Read the model definition and answer for the solid it produces. Units are mm, in the model's axes. A direction names the side the tool comes from. Coordinates: 2 decimals unless noted, no trailing zeros. Order: outer loops, then holes, each group sorted by start corner. A loop starts at its lowest first (then second) coordinate and runs counter-clockwise, first axis right, second up. Notation, with made-up numbers: (3.5, 44.5) - (39.5, 44.5) arc R15 ccw to (39.5, 48.5) - close; hole circle Ø9 at (76.5, 46). An arc over 180 degrees is marked (long way). Use one line per item in the form item = value.
```python
from build123d import *

# Parameters (mm, degrees)
SKETCH1_W           = 25.4
SKETCH1_H           = 25.4
BOSS_EXTRUDE1_DEPTH = 114.3
SKETCH3_W           = 22.098
SKETCH3_H           = 22.098
CUT_EXTRUDE1_DEPTH  = 130.139939168
SKETCH4_W           = 20.6248
SKETCH4_H           = 50.8
CUT_EXTRUDE2_DEPTH  = 128.825773065
SKETCH5_R           = 3.302
CUT_EXTRUDE3_DEPTH  = 122.212646323


with BuildPart() as part:
    # Sketch1 → Boss-Extrude1 (new body)
    with BuildSketch(Plane.XY):
        with Locations((-38.581363669, -18.650528362)):
            Rectangle(SKETCH1_W, SKETCH1_H)
    extrude(amount=BOSS_EXTRUDE1_DEPTH)

    # Sketch3 → Cut-Extrude1 (cut, through all)
    with BuildSketch(Plane.XY.offset(114.3)):
        with Locations((-38.581363669, -18.650528362)):
            Rectangle(SKETCH3_W, SKETCH3_H)
    extrude(amount=-CUT_EXTRUDE1_DEPTH, mode=Mode.SUBTRACT)

    # Sketch4 → Cut-Extrude2 (cut, through all)
    with BuildSketch(Plane(origin=(0, -5.950528362, 0), x_dir=(1, 0, 0), z_dir=(0, 1, 0))):
        with Locations((-38.581363669, -114.3)):
            Rectangle(SKETCH4_W, SKETCH4_H)
    extrude(amount=-CUT_EXTRUDE2_DEPTH, mode=Mode.SUBTRACT)

    # Sketch5 → Cut-Extrude3 (cut, through all)
    with BuildSketch(Plane.ZY.offset(51.281363669)):
        with Locations((104.775, -19.04458559)):
            Circle(SKETCH5_R)
    extrude(amount=-CUT_EXTRUDE3_DEPTH, mode=Mode.SUBTRACT)


solid = part.part
```
(1) Which of the six approach directions +Z, -Z, +X, -X, +Y, -Y give full straight-line access (tool end or side, diameter ignored) to faces 4 (the flat face through (-39, -29.7, 45)), 5 (the flat face through (-51.281, -19, 56))?
Answer list:
face_4 = +Z, -Z
face_5 = +Z, -Z, -X, +Y, -Y
(2) Straight lines are drawn through the part: L1, parallel to Y at x = -49, z = 67; L2, parallel to X at y = -11, z = 10.5. For each, find the intervals that lie inside material, in ascending order.
Answer list:
L1 = -31.35 to -29.7, -7.6 to -5.95
L2 = -51.28 to -49.63, -27.53 to -25.88
(3) Section A-A, the plane x = -47.75 is taken. Write down the section's boundary in (y, z), then the cut area to 3 significant figures.
Answer list:
outline = (-31.35, 0) - (-29.7, 0) - (-29.7, 88.9) - (-31.35, 88.9) - close; (-7.6, 0) - (-5.95, 0) - (-5.95, 88.9) - (-7.6, 88.9) - close
area = 294 mm2
(4) Section C-C, the plane z = 27 is taken. Write down the section's boundary in (x, y), then the cut area to 3 significant figures.
Answer list:
outline = (-51.28, -31.35) - (-25.88, -31.35) - (-25.88, -5.95) - (-51.28, -5.95) - close; hole (-49.63, -29.7) - (-27.53, -29.7) - (-27.53, -7.6) - (-49.63, -7.6) - close
area = 157 mm2
(5) Section B-B, the plane y = -13.5 is taken. Write down the section's boundary in (x, z).
Answer list:
outline = (-51.28, 0) - (-49.63, 0) - (-49.63, 114.3) - (-51.28, 114.3) - close; (-27.53, 0) - (-25.88, 0) - (-25.88, 114.3) - (-27.53, 114.3) - close
(6) Given pin 1 Ø1.8 at (x, y) = (-38, -7) entering from +Z, flat-ended and moving along its own axis, determine where the tip first touches the part or whether it passes through.
Answer list:
pin_1 = 88.9
(7) The mould has two halves that part along X. Classify faces 1 (the flat face through (-39, -5.951, 44)), 2 (the flat face through (-25.881, -19, 56)), 3 (the flat face through (-27.532, -19, 58)): +X half, -X half, draft (parallel to the pull), parting line (faces both ways), or undercut.
Answer list:
face_1 = draft
face_2 = +X half
face_3 = undercut
